The listing builds one solid part. Answer for the finished solid, in the listing's coordinates (mm). Face numbers are marked on the shaded views. A direction names the side the tool comes from. Coordinates: 2 decimals unless noted, no trailing zeros. Order: outer loops, then holes, each group sorted by start corner. A loop starts at its lowest first (then second) coordinate and runs counter-clockwise, first axis right, second up. Notation, with made-up numbers: (39.5, 36.25) - (71.5, 36.25) arc R26 cw to (71.5, 56.25) - close; hole circle Ø1 at (58.25, -10). An arc over 180 degrees is marked (long way). Use a Markdown table: item, result. Add a question column.
Item 1: The mould has two halves that part along X. Classify the marked faces 1, 2 and 3: released by +X, released by -X, zero draft, split by the parting line, or undercut.
Item 2: Flat-ended cylindrical pins translate along their axes: P1, Ø6, axis at x = -10.5, y = -17, coming from the -Z side; P2, Ø6, axis at x = 42, y = -24.5, coming from the -Z side; P3, Ø6, axis at x = 28, z = -6.5, coming from the -Y side. Find the tip coordinate at first contact, or state that the pin passes through.
Item 3: The part is cut by section B-B, the plane y = -44. Give the vertices of the cut face in (x, z), then the cut area to 3 significant figures.
Item 4: The part is cut by section D-D, the plane y = -20. State how many separate pieces and enclosed holes the cut face has, then the cut area to 3 significant figures.
Item 5: For the marked faces 4 and 5, determine the directions among +Z, -Z, +X, -X, +Y, -Y from which every point of the face is accessible in a straight line to the end or side of a thin tool.
Item 6: The part is cut by section A-A, the plane x = 0. Give the vertices of the cut face in (y, z).
Item 7: The part is cut by section C-C, the plane x = -20. Give the vertices of the cut face in (y, z), then the cut area to 3 significant figures.
Item 8: Find the intervals of material crossed by line 1 along Y through (x, z) = (0, -1.25); line 2 along Z through (x, y) = (35, -10.5); line 3 along X through (y, z) = (-37, 3.25), in increasing order.
from build123d import *

# Parameters (mm, degrees)
SKETCH1_R           = 5.05
BOSS_EXTRUDE1_DEPTH = 5
BOSS_EXTRUDE2_START = 5
BOSS_EXTRUDE2_DEPTH = 5
BOSS_EXTRUDE4_DEPTH = 2
CUT_EXTRUDE1_START  = -3
SKETCH6_R           = 9.5
SKETCH6_R_2         = 5.05
CUT_EXTRUDE1_DEPTH  = 3
SKETCH7_R           = 2.5
CUT_EXTRUDE2_DEPTH  = 74.87151007
SKETCH8_R           = 5
BOSS_EXTRUDE5_DEPTH = 3
CUT_EXTRUDE3_DEPTH  = 3
SKETCH10_W          = 8.596273884
SKETCH10_H          = 2
CUT_REVOLVE1_ANGLE  = 180


with BuildPart() as part:
    # Sketch1 → Boss-Extrude1 (new body)
    with BuildSketch(Plane.XY):
        with BuildLine():
            Line((-52, 0), (52, 0))
            ThreePointArc((52, 0), (0, -52), (-52, 0))
        make_face()
        with Locations((20, -20)):
            Circle(SKETCH1_R, mode=Mode.SUBTRACT)
    extrude(amount=-BOSS_EXTRUDE1_DEPTH)

    # Sketch2 → Boss-Extrude2 (add)
    with BuildSketch(Plane.XY.offset(BOSS_EXTRUDE2_START)):
        with BuildLine():
            Line((52, 0), (-52, 0))
            ThreePointArc((-52, 0), (0, -52), (52, 0))
        make_face()
        with BuildLine():
            Line((49.959983987, -2), (-49.959983987, -2))
            ThreePointArc((-49.959983987, -2), (0, -50), (49.959983987, -2))
        make_face(mode=Mode.SUBTRACT)
    extrude(amount=-BOSS_EXTRUDE2_DEPTH)

    # Sketch5 → Boss-Extrude4 (add)
    with BuildSketch(Plane(origin=(0, 0, -5), x_dir=(-1, 0, 0), z_dir=(0, 0, -1))):
        with BuildLine():
            ThreePointArc((-49.323463146, -16.468029126), (-45.033320997, -26), (-38.923463146, -34.481357524))
            Line((-38.923463146, -34.481357524), (-37.426406871, -33.155151466))
            ThreePointArc((-37.426406871, -33.155151466), (-43.301270189, -25), (-47.426406871, -15.83464339))
            Line((-47.426406871, -15.83464339), (-49.323463146, -16.468029126))
        make_face()
        with BuildLine():
            Line((10.4, -50.94938665), (10, -48.989794856))
            ThreePointArc((10, -48.989794856), (0, -50), (-10, -48.989794856))
            Line((-10, -48.989794856), (-10.4, -50.94938665))
            ThreePointArc((-10.4, -50.94938665), (0, -52), (10.4, -50.94938665))
        make_face()
        with BuildLine():
            Line((37.426406871, -33.155151466), (38.923463146, -34.481357524))
            ThreePointArc((38.923463146, -34.481357524), (45.033320997, -26), (49.323463146, -16.468029126))
            Line((49.323463146, -16.468029126), (47.426406871, -15.83464339))
            ThreePointArc((47.426406871, -15.83464339), (43.301270189, -25), (37.426406871, -33.155151466))
        make_face()
    extrude(amount=BOSS_EXTRUDE4_DEPTH)

    # Sketch6 → Cut-Extrude1 (cut)
    with BuildSketch(Plane(origin=(0, 0, -5), x_dir=(-1, 0, 0), z_dir=(0, 0, -1)).offset(CUT_EXTRUDE1_START)):
        with Locations((0, -20)):
            Circle(SKETCH6_R)
        with Locations(Location((-20, -20, 0), (0, 0, 180))):
            Circle(SKETCH6_R_2)
    extrude(amount=CUT_EXTRUDE1_DEPTH, mode=Mode.SUBTRACT)

    # Sketch7 → Cut-Extrude2 (cut, through all)
    with BuildSketch(Plane(origin=(0, 0, -2), x_dir=(-1, 0, 0), z_dir=(0, 0, -1))):
        with Locations((0, -20)):
            Circle(SKETCH7_R)
    extrude(amount=-CUT_EXTRUDE2_DEPTH, mode=Mode.SUBTRACT)

    # Sketch8 → Boss-Extrude5 (add)
    with BuildSketch(Plane(origin=(0, 0, -5), x_dir=(-1, 0, 0), z_dir=(0, 0, -1))):
        with Locations(Location((20, -20, 0), (0, 0, 180))):
            Circle(SKETCH8_R)
    extrude(amount=BOSS_EXTRUDE5_DEPTH)

    # Sketch9 → Cut-Extrude3 (cut)
    # profile 1 of 2: a face of its own
    with BuildSketch(Plane.XY.offset(5)):
        with BuildLine():
            Line((50.990195136, -1), (-50.990195136, -1))
            ThreePointArc((-50.990195136, -1), (0, -51), (50.990195136, -1))
        make_face()
        with BuildLine():
            ThreePointArc((49.959983987, -2), (0, -50), (-49.959983987, -2))
            Line((-49.959983987, -2), (49.959983987, -2))
        make_face(mode=Mode.SUBTRACT)
    # profile 2 of 2: a face of its own
    with BuildSketch(Plane.XY.offset(5)):
        with BuildLine():
            Line((-49.959983987, -2), (49.959983987, -2))
            ThreePointArc((49.959983987, -2), (0, -50), (-49.959983987, -2))
        make_face()
    extrude(amount=-CUT_EXTRUDE3_DEPTH, mode=Mode.SUBTRACT)

    # Sketch10 → Cut-Revolve1 (revolve, cut)
    with BuildSketch(Plane(origin=(0, 0, 0), x_dir=(1, 0, 0), z_dir=(0, 1, 0))):
        with Locations((54.298136942, 2)):
            Rectangle(SKETCH10_W, SKETCH10_H)
    revolve(axis=Axis((0, 0, -7.000025), (0, 0, -1)), revolution_arc=CUT_REVOLVE1_ANGLE, mode=Mode.SUBTRACT)


solid = part.part
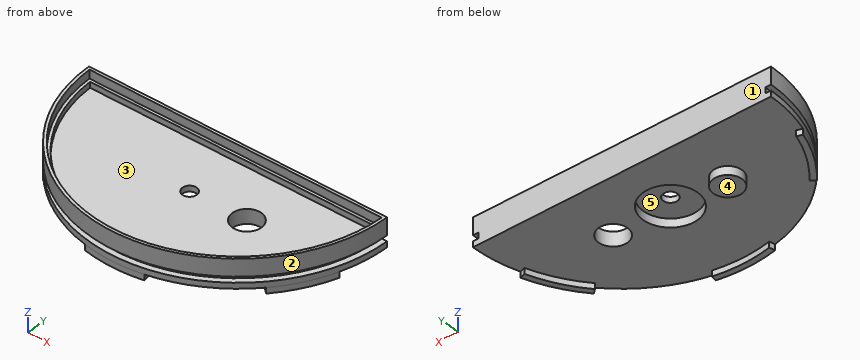
Solution:
| question | item | result |
|---|---|---|
| 1 | face 1 | zero draft |
| 1 | face 2 | split by the parting line |
| 1 | face 3 | undercut |
| 2 | P1 | stops at z = -5 |
| 2 | P2 | stops at z = -7 |
| 2 | P3 | stops at y = -45.37 |
| 3 | outline | (-27.71, -5) - (27.71, -5) - (27.71, -3) - (23.75, -3) - (23.75, -1) - (27.71, -1) - (27.71, 5) - (25.79, 5) - (25.79, 2) - (23.75, 2) - (23.75, 0) - (-23.75, 0) - (-23.75, 2) - (-25.79, 2) - (-25.79, 5) - (-27.71, 5) - (-27.71, -1) - (-23.75, -1) - (-23.75, -3) - (-27.71, -3) - close |
| 3 | area | 289 mm2 |
| 4 | separate pieces | 3 |
| 4 | enclosed holes | 0 |
| 4 | area | 408 mm2 |
| 5 | face 4 | -Z, +X, -X, +Y, -Y |
| 5 | face 5 | -Z |
| 6 | outline | (-52, -7) - (-50, -7) - (-50, -5) - (-29.5, -5) - (-29.5, -2) - (-22.5, -2) - (-22.5, 0) - (-50, 0) - (-50, 2) - (-51, 2) - (-51, 5) - (-52, 5) - (-52, -1) - (-50, -1) - (-50, -3) - (-52, -3) - close; (-17.5, -2) - (-10.5, -2) - (-10.5, -5) - (0, -5) - (0, 5) - (-1, 5) - (-1, 2) - (-2, 2) - (-2, 0) - (-17.5, 0) - close |
| 7 | outline | (-48, -5) - (-25, -5) - (-25, -8) - (-15, -8) - (-15, -5) - (0, -5) - (0, 5) - (-1, 5) - (-1, 2) - (-2, 2) - (-2, 0) - (-45.83, 0) - (-45.83, 2) - (-46.91, 2) - (-46.91, 5) - (-48, 5) - (-48, -1) - (-45.83, -1) - (-45.83, -3) - (-48, -3) - close |
| 7 | area | 280 mm2 |
| 8 | line 1 | y = -50 to -22.5, -17.5 to 0 |
| 8 | line 2 | z = -5 to 0 |
| 8 | line 3 | x = -36.54 to -35.1, 35.1 to 36.54 |
